```python
from build123d import *

# Parameters (mm, degrees)
SKETCH8_W           = 144
SKETCH8_H           = 50
SKETCH8_R           = 6
BOSS_EXTRUDE5_DEPTH = 37.5
SKETCH9_W           = 51
SKETCH9_H           = 38
CUT_EXTRUDE1_DEPTH  = 157.978501713
CUT_EXTRUDE2_DEPTH  = 116.364639296


with BuildPart() as part:
    # Sketch8 → Boss-Extrude5 (new, symmetric)
    with BuildSketch(Plane(origin=(0, 0, 0), x_dir=(0, 0, -1), z_dir=(1, 0, 0))):
        with Locations((0, 25)):
            Rectangle(SKETCH8_W, SKETCH8_H)
        with Locations((-19, 31)):
            Circle(SKETCH8_R, mode=Mode.SUBTRACT)
        with Locations((19, 31)):
            Circle(SKETCH8_R, mode=Mode.SUBTRACT)
    extrude(amount=BOSS_EXTRUDE5_DEPTH, both=True)

    # Sketch9 → Cut-Extrude1 (cut, through all)
    with BuildSketch(Plane.XY.offset(72)):
        with Locations((0, 31)):
            Rectangle(SKETCH9_W, SKETCH9_H)
    extrude(amount=-CUT_EXTRUDE1_DEPTH, mode=Mode.SUBTRACT)

    # Sketch10 → Cut-Extrude2 (cut, through all)
    with BuildSketch(Plane(origin=(37.5, 0, 0), x_dir=(0, 0, -1), z_dir=(1, 0, 0))):
        with BuildLine():
            Line((-72, 50), (-34, 50))
            ThreePointArc((-34, 50), (-47.460763972, 25.460763972), (-72, 12))
            Line((-72, 12), (-72, 50))
        make_face()
        with BuildLine():
            Line((72, 50), (34, 50))
            ThreePointArc((34, 50), (47.460763972, 25.460763972), (72, 12))
            Line((72, 12), (72, 50))
        make_face()
    extrude(amount=-CUT_EXTRUDE2_DEPTH, mode=Mode.SUBTRACT)


solid = part.part
```
Geometry: final body of the model. Coordinates: model frame, mm. A direction names the side the tool comes from. Coordinates: 2 decimals unless noted, no trailing zeros. Order: outer loops, then holes, each group sorted by start corner. A loop starts at its lowest first (then second) coordinate and runs counter-clockwise, first axis right, second up. Notation, with made-up numbers: M 34,49.25 L 51,49.25 A13 cw 51,56.25 Z; hole C -2,45.5 d1. An arc over 180 degrees is marked long. Answer as CSV lines item,"result".
Q1. Section D-D on z = -18. Return the cut outline in (x, y), and give its area (3 significant figures).
Answers:
outline,"M -37.5,0 L 37.5,0 L 37.5,25.08 L 25.5,25.08 L 25.5,12 L -25.5,12 L -25.5,25.08 L -37.5,25.08 Z; M -37.5,36.92 L -25.5,36.92 L -25.5,50 L -37.5,50 Z; M 25.5,36.92 L 37.5,36.92 L 37.5,50 L 25.5,50 Z"
area,"1,530 mm^2"
Q2. First-contact query: P1, Ø1.5, axis at x = -24, z = -23.5, coming from the +Y side; P2, Ø1.5, axis at x = -27, y = 36.5, coming from the +Z side. Flat tips, straight axial feed; report the tip coordinate or a pass-through.
Answers:
P1,"stops at y = 12"
P2,"stops at z = 39.55"
Q3. Section B-B on z = 19. Return the cut outline in (x, y), and give its area (3 significant figures).
Answers:
outline,"M -37.5,0 L 37.5,0 L 37.5,25 L 25.5,25 L 25.5,12 L -25.5,12 L -25.5,25 L -37.5,25 Z; M -37.5,37 L -25.5,37 L -25.5,50 L -37.5,50 Z; M 25.5,37 L 37.5,37 L 37.5,50 L 25.5,50 Z"
area,"1,520 mm^2"
Q4. Draft query along Y for faces 1 (the flat face through (1, 6, 72)), 2 (the cylindrical face through (31.416, 25.143, 20.301)), 3 (the cylindrical face through (31.584, 25.743, 47.181)). Return one class per face: pulls with the +Y half, pulls with the -Y half, needs draft (parallel to the pull), parting line crosses it, or undercut.
Answers:
face 1,"needs draft"
face 2,"undercut"
face 3,"pulls with the +Y half"
Q5. Line query: probe 1 along X at (y, z) = (46, -16.5); probe 2 along Y at (x, z) = (-33, 19); probe 3 along Z at (x, y) = (-32.5, 31). Output: solid intervals per line, ascending. Write a range as [from, to].
Answers:
probe 1,"x = [-37.5, -25.5], [25.5, 37.5]"
probe 2,"y = [0, 25], [37, 50]"
probe 3,"z = [-42.68, -25], [-13, 13], [25, 42.68]"
Q6. Set-up query: faces 4 (the flat face through (1, 0, 1)), 5 (the flat face through (0, 12, 1)). Return all of +Z, -Z, +X, -X, +Y, -Y with unobstructed straight access to the full face (end or side cutting, diameter ignored); none if empty.
Answers:
face 4,"+Z, -Z, +X, -X, -Y"
face 5,"+Z, -Z, +Y"
Q7. Section A-A on y = 31. Return the cut outline in (x, z).
Answers:
outline,"M -37.5,-42.68 L -25.5,-42.68 L -25.5,-25 L -37.5,-25 Z; M -37.5,-13 L -25.5,-13 L -25.5,13 L -37.5,13 Z; M -37.5,25 L -25.5,25 L -25.5,42.68 L -37.5,42.68 Z; M 25.5,-42.68 L 37.5,-42.68 L 37.5,-25 L 25.5,-25 Z; M 25.5,-13 L 37.5,-13 L 37.5,13 L 25.5,13 Z; M 25.5,25 L 37.5,25 L 37.5,42.68 L 25.5,42.68 Z"
Q8. Section C-C on x = 20. Return the cut outline in (y, z), and give its area (3 significant figures).
Answers:
outline,"M 0,-72 L 12,-72 L 12,72 L 0,72 Z"
area,"1,730 mm^2"
